from build123d import *

# Parameters (mm, degrees)
F0_W     = 192.96
F0_H     = 110.76
F1_DEPTH = 3
F2_R     = 7.5


with BuildPart() as f1:
    # F0 (on Front) → F1 (new body)
    with BuildSketch(Plane.XZ):
        with BuildLine():
            ThreePointArc((105, 56.4), (102.803301, 61.703301), (97.5, 63.9))
            Line((97.5, 63.9), (-97.5, 63.9))
            ThreePointArc((-97.5, 63.9), (-102.803301, 61.703301), (-105, 56.4))
            Line((-105, 56.4), (-105, -56.4))
            ThreePointArc((-105, -56.4), (-102.803301, -61.703301), (-97.5, -63.9))
            Line((-97.5, -63.9), (97.5, -63.9))
            ThreePointArc((97.5, -63.9), (102.803301, -61.703301), (105, -56.4))
            Line((105, -56.4), (105, 56.4))
        make_face()
        Rectangle(F0_W, F0_H, mode=Mode.SUBTRACT)
    extrude(amount=F1_DEPTH)

    # F2
    f2_edges = [f1.edges().sort_by_distance(p)[0] for p in [
        (96.48, -1.5, 55.38),
        (-96.48, -1.5, 55.38),
        (-96.48, -1.5, -55.38),
        (96.48, -1.5, -55.38),
    ]]
    fillet(f2_edges, radius=F2_R)


solid = f1.part
Could you check a few things on this model? Use its own coordinates, in mm. A direction names the side the tool comes from. Coordinates: 2 decimals unless noted, no trailing zeros. Order: outer loops, then holes, each group sorted by start corner. A loop starts at its lowest first (then second) coordinate and runs counter-clockwise, first axis right, second up.
Q1. Thinking about a two-plate mould opening in X: for faces 3 (the cylindrical face through (-94.225, -1.521, -53.241)), 4 (the cylindrical face through (-102.745, -1.479, 61.761)), 5 (the flat face through (-8, -3, -57)), which applies, released by +X, released by -X, zero draft, split by the parting line, or undercut?
Q2. Please list where these lines run through material, in increasing order: L1, parallel to Z at x = 8, y = -0.7; L2, parallel to X at y = -0.85, z = -24.5; L3, parallel to X at y = -0.4, z = 50.5.
Q3. Suppose I cut it at A-A on y = -1.45. Please give me the cut outline in (x, z).
Q4. Which directions (+Z, -Z, +X, -X, +Y, -Y) give clear straight access to the entire face, cutting with the end or side of a thin tool? Please do faces 1 (the cylindrical face through (102.745, -1.479, -61.761)), 2 (the cylindrical face through (94.225, -1.521, -53.241)).
Q5. Suppose I cut it at C-C on z = 2. Please give me the cut outline in (x, y).
Q6. Suppose I cut it at B-B on x = -10. Please give me the cut outline in (y, z), and give its area (3 significant figures).
Answer:
1. face 3: undercut
1. face 4: released by -X
1. face 5: zero draft
2. L1: z = -63.9 to -55.38, 55.38 to 63.9
2. L2: x = -105 to -96.48, 96.48 to 105
2. L3: x = -105 to -96.01, 96.01 to 105
3. outline: (-105, -56.4) arc R7.5 ccw to (-97.5, -63.9) - (97.5, -63.9) arc R7.5 ccw to (105, -56.4) - (105, 56.4) arc R7.5 ccw to (97.5, 63.9) - (-97.5, 63.9) arc R7.5 ccw to (-105, 56.4) - close; hole (-96.48, -47.88) arc R7.5 ccw to (-88.98, -55.38) - (88.98, -55.38) arc R7.5 ccw to (96.48, -47.88) - (96.48, 47.88) arc R7.5 ccw to (88.98, 55.38) - (-88.98, 55.38) arc R7.5 ccw to (-96.48, 47.88) - close
4. face 1: -Z, +X, +Y, -Y
4. face 2: +Y, -Y
5. outline: (-105, -3) - (-96.48, -3) - (-96.48, 0) - (-105, 0) - close; (96.48, -3) - (105, -3) - (105, 0) - (96.48, 0) - close
6. outline: (-3, -63.9) - (0, -63.9) - (0, -55.38) - (-3, -55.38) - close; (-3, 55.38) - (0, 55.38) - (0, 63.9) - (-3, 63.9) - close
6. area: 51.1 mm2
